Autodesk Inventor part; units mm, degrees
ref_plane "РабПлоскость2" through (1.8806, 0, -2.7594) normal (-1, 0, 0) x (0, 0, 1)
ref_plane "РабПлоскость3" through (-4.0194, 25.1, -3.1709) normal (0, -1, 0) x (1, 0, 0)
ref_plane "YZ Plane" through (0, 0, 0) normal (1, 0, 0) x (0, 1, 0)
sketch "Эскиз1" plane through (0, 0, 0) normal (0, 1, 0) x (-1, 0, 0)
  arc A0 (4.0194, -3.1709) -> (-7.7806, -3.1709) centre (-1.8806, -45.2594) ccw
  line L0 (-7.7806, -3.1709) -> (-7.7806, 2.8291)
  line L1 (-7.7806, 2.8291) -> (4.0194, 2.8291)
  line L2 (4.0194, 2.8291) -> (4.0194, -3.1709)
  point P0 (0, -39)
  dimension "d1" = 6
  dimension "d12" = 11.8
extrude "Выдавливание1" add sketch "Эскиз1" along normal blind 50.2
sketch "Эскиз4" plane through (0, 0, 0) normal (0, -1, 0) x (1, 0, 0)
  arc A0 (7.7806, -3.1709) -> (-4.0194, -3.1709) centre (1.8806, -45.2594) ccw
  line L0 (1.8806, -2.7594) -> (-4.0194, -2.7594)
  line L1 (-4.0194, -3.1709) -> (-4.0194, 2.8291)
  line L2 (-4.0194, 2.8291) -> (-19.0194, 2.8291)
  line L3 (-19.0194, 2.8291) -> (-19.0194, -2.7594)
  line L4 (-19.0194, -2.7594) -> (-4.0194, -2.7594)
  line L5 (-4.0194, -2.7594) -> (-4.0194, 2.8291)
  line L6 (7.7806, 2.8291) -> (7.7806, -3.1709)
  line L7 (7.7806, 2.8291) -> (22.7806, 2.8291)
  line L8 (22.7806, 2.8291) -> (22.7806, -2.7594)
  line L9 (22.7806, -2.7594) -> (7.7806, -2.7594)
  line L10 (7.7806, -2.7594) -> (7.7806, 2.8291)
  point P0 (0, 0)
  dimension "d13" = 15
  dimension "d16" = 15
extrude "Выдавливание4" add sketch "Эскиз4" against normal up to surface (50.2 mm away) contours L4 L3 L2 L1 | L6 L7 L8 L9
sketch "Эскиз5" plane through (0, 0, 0) normal (0, -1, 0) x (1, 0, 0)
  line L0 (22.7806, 2.8291) -> (-19.0194, 2.8291)
  line L1 (1.8806, 2.8291) -> (1.8806, -0.1709)
  line L2 (1.8806, -0.1709) -> (-8.1194, -0.1709)
  line L3 (-8.1194, -0.1709) -> (11.8806, -0.1709)
  circle A0 centre (-8.1194, -0.1709) radius 1.5
  circle A1 centre (11.8806, -0.1709) radius 1.5
  point P0 (0, 0)
  dimension "d17" = 3
  dimension "d18" = 10
  dimension "d19" = 20
  dimension "d20" = 3
  dimension "d21" = 3
extrude "Выдавливание5" cut sketch "Эскиз5" against normal blind 10
sketch "Эскиз6" plane through (0, 50.2, 0) normal (0, 1, 0) x (1, 0, 0)
  circle A0 centre (-8.1194, 0.1709) radius 1.5
  circle A1 centre (-8.1194, 0.1709) radius 1.5
  circle A2 centre (11.8806, 0.1709) radius 1.5
  circle A3 centre (11.8806, 0.1709) radius 1.5
  point P0 (0, 0)
extrude "Выдавливание6" cut sketch "Эскиз6" against normal blind 10
sketch "Эскиз7" plane through (-19.0194, 0, 2.8291) normal (0, 0, 1) x (1, 0, 0)
  line L0 (0, 0) -> (0, 50.2)
  line L1 (0, 0) -> (3, 0)
  line L2 (3, 0) -> (3, 3)
  line L3 (3, 3) -> (0, 3)
  line L4 (0, 3) -> (0, 0)
  circle A0 centre (3, 3) radius 1.5
  point P0 (19.0194, 0)
  dimension "d26" = 3
  dimension "d27" = 3
  dimension "d28" = 3
extrude "Выдавливание7" cut sketch "Эскиз7" against normal blind 10 contours A0 L2 L3 | L3 L2 A0
sketch "Эскиз8" plane through (-4.0194, 0, -2.7594) normal (0, 0, -1) x (-1, 0, 0)
  circle A0 centre (12, 3) radius 1.5
  line L0 (13.85, 3) -> (12.925, 1.3979)
  line L1 (12.925, 1.3979) -> (11.075, 1.3979)
  line L2 (11.075, 1.3979) -> (10.15, 3)
  line L3 (10.15, 3) -> (11.075, 4.6021)
  line L4 (11.075, 4.6021) -> (12.925, 4.6021)
  line L5 (12.925, 4.6021) -> (13.85, 3)
  point P0 (-4.0194, 0)
  dimension "d31" = 3.7
extrude "Выдавливание8" cut sketch "Эскиз8" against normal blind 2.8 contours A0 | L0 L1 L2 L3 L4 L5
ref_plane "РабПлоскость2" through (1.8806, 0, -2.7594) normal (-1, 0, 0) x (0, 0, 1)
ref_plane "РабПлоскость3" through (-4.0194, 25.1, -3.1709) normal (0, -1, 0) x (1, 0, 0)
mirror "Зеркальное отражение2" about plane through (1.8806, 0, -2.7594) normal (-1, 0, 0) of "Выдавливание8", "Выдавливание7"
mirror "Зеркальное отражение3" about plane through (-4.0194, 25.1, -3.1709) normal (0, -1, 0) of "Выдавливание8", "Выдавливание7", "Зеркальное отражение2"
sketch "Эскиз9" plane through (-19.0194, 0, 2.8291) normal (0, 0, 1) x (1, 0, 0)
  circle A0 centre (38.8, 47.2) radius 1.5
  circle A1 centre (3, 47.2) radius 1.5
  circle A2 centre (38.8, 3) radius 1.5
  circle A3 centre (3, 3) radius 1.5
  line L0 (41.8, 0) -> (0, 0)
  line L1 (41.8, 0) -> (41.8, 50.2)
  line L2 (41.8, 50.2) -> (0, 50.2)
  line L3 (0, 0) -> (0, 50.2)
  point P0 (19.0194, 0)
properties part number "joint3_rot_con" material "Пластик АБС"
For this review, take the finished solid that the model builds, in its own axes (mm). A direction names the side the tool comes from. Give positions to 0.01 mm unless a question says otherwise; leave off trailing zeros. Order: outer loops, then holes, each group sorted by start corner. A loop starts at its lowest first (then second) coordinate and runs counter-clockwise, first axis right, second up. Notation, with made-up numbers: M 4.25,80.5 L 48.25,80.5 A27 cw 48.25,116.5 Z; hole C -31,70.5 d3. An arc over 180 degrees is marked long. Answer in a Markdown table with one row per item. Add a question column.
(1) For pin 1 (0.9 mm diameter, centred on x = -8.5, z = 0.5, fed in from -Y); pin 2 (7.5 mm diameter, centred on x = -11.5, y = 17.5, fed in from -Z), all flat-tipped, find the tip position at first contact; note any pin that passes through.
(2) Consider section A-A on y = 33.5. State the section outline as (x, z) points.
(3) Wall thickness on probe 1 along Y at (x, z) = (-15, 1.75); probe 2 along Z at (x, y) = (-8, 3); probe 3 along X at (y, z) = (3, -0.15): over which ranges is each line inside the solid? List them lowest first. Write a range as [from, to].
(4) Consider section C-C on z = -0.8. Give the number of separate pieces and of enclosed holes in the cut face, and give its area (3 significant figures).
(5) For faces 5 (the face through (15, 25, -2.759)), 6 (the face through (-6.734, 45.27, 0.404)), 7 (the face through (-14.638, 2.188, -1.379)), 8 (the face through (-8, 10, 0)), list the 3-axis set-ups (+Z, -Z, +X, -X, +Y, -Y) from which the entire face can be reached by the end or side of a thin tool; tool diameter is ignored.
(6) Mouldability with a two-part tool opening along X and no side actions: class faces 1 (the face through (22.781, 25, 0)), 2 (the face through (18.4, 48.01, -1.38)), 3 (the face through (-19.019, 25, 0)), 4 (the face through (21.162, 46.388, -1.379)) as +X half, -X half, draft (parallel to the pull), parting line (faces both ways), or undercut.
(7) Consider section B-B on x = 16.5. State the section outline as (y, z) points, and give its area (3 significant figures).
Evaluation:
| question | item | result |
|---|---|---|
| 1 | pin 1 | stops at y = 10 |
| 1 | pin 2 | stops at z = -2.76 |
| 2 | outline | M -19.02,-2.76 L -4.02,-2.76 L -4.02,-3.17 A42.5 cw 7.78,-3.17 L 7.78,-2.76 L 22.78,-2.76 L 22.78,2.83 L -19.02,2.83 Z |
| 3 | probe 1 | y = [0, 1.9], [4.1, 46.1], [48.3, 50.2] |
| 3 | probe 2 | z = [-2.76, -1.67], [1.32, 2.83] |
| 3 | probe 3 | x = [-19.02, -17.87], [-14.17, -9.62], [-6.62, 10.38], [13.38, 17.93], [21.63, 22.78] |
| 4 | separate pieces | 1 |
| 4 | enclosed holes | 4 |
| 4 | area | 1,950 mm^2 |
| 5 | face 5 | -Z, +X, +Y, -Y |
| 5 | face 6 | +Y |
| 5 | face 7 | -Z |
| 5 | face 8 | -Y |
| 6 | face 1 | +X half |
| 6 | face 2 | undercut |
| 6 | face 3 | -X half |
| 6 | face 4 | undercut |
| 7 | outline | M 0,-2.76 L 50.2,-2.76 L 50.2,2.83 L 0,2.83 Z |
| 7 | area | 281 mm^2 |
